Work out the finished part from the listing and answer in its coordinate system (mm). Give positions to 0.01 mm unless a question says otherwise; leave off trailing zeros. Write each loop counter-clockwise with the first axis right and the second up, starting at its lowest first coordinate (ties: lowest second). Pieces come first, ordered by that corner, then holes.
1) Find section D-D (z = 51.5). Determine the outline of the cut face in (x, y).
2) Given pin 1 Ø6.5 at (y, z) = (20, 62.5) entering from +X; pin 2 Ø5 at (x, z) = (-11, 45.5) entering from -Y; pin 3 Ø6 at (y, z) = (25.5, 18.5) entering from +X, each flat-ended and moving along its own axis, determine where each tip first touches the part or whether it passes through.
3) Determine the mould class of faces 1 (the face through (0, 0, 70)), 2 (the face through (-0.195, 31.487, 35.49)), 3 (the face through (-13.366, -0.49, 3.581)) for opening direction X: pulls with the +X half, pulls with the -X half, needs draft (parallel to the pull), parting line crosses it, or undercut.
4) Find section C-C (x = 6). Determine the outline of the cut face in (y, z).
5) Find section A-A (z = 66). Determine the outline of the cut face in (x, y), plus the area to 3 significant figures.
6) Find section B-B (y = -30). Determine the outline of the cut face in (x, z).
7) Straight lines are drawn through the part: probe 1 along Y at (x, z) = (-20, 53); probe 2 along Y at (x, z) = (-12, 62.5); probe 3 along Y at (x, z) = (0.5, 43.5). For each, find the intervals that lie inside material, in ascending order.
```python
from build123d import *

# Parameters (mm, degrees)
F0_R          = 35
F1_DEPTH      = 70
F3_DEPTH      = 35.001
F3_DEPTH_BACK = 35.001
F4_R          = 2.5
F5_DEPTH      = 35.001
F5_DEPTH_BACK = 35.001
F8_R          = 0.5
F9_DEPTH      = 20
F10_R         = 1.5
F11_DEPTH     = 70.0010001


with BuildPart() as f1:
    # F0 (on Top) → F1 (new body)
    with BuildSketch(Plane.XY):
        Circle(F0_R)
    extrude(amount=F1_DEPTH)

    # F2 (on Front) → F3 (cut, two sides)
    with BuildSketch(Plane.XZ) as f3_sk:
        Polygon((-50, 0), (0, 0), (-50, 13.3974596216), align=None)
        Polygon((50, 23.3153829077), (0, 0), (50, 0), align=None)
    extrude(amount=-F3_DEPTH, mode=Mode.SUBTRACT)
    extrude(f3_sk.sketch, amount=F3_DEPTH_BACK, mode=Mode.SUBTRACT)

    # F4 (on Right) → F5 (cut, two sides)
    with BuildSketch(Plane.YZ) as f5_sk:
        with Locations((-20, 62.5)):
            Circle(F4_R)
        with Locations((20, 62.5)):
            Circle(F4_R)
    extrude(amount=-F5_DEPTH, mode=Mode.SUBTRACT)
    extrude(f5_sk.sketch, amount=F5_DEPTH_BACK, mode=Mode.SUBTRACT)

    # F6 (on Front) → F7 (revolve, cut)
    with BuildSketch(Plane.XZ):
        with BuildLine():
            Line((0, 15), (0, 55))
            ThreePointArc((0, 55), (-20, 35), (0, 15))
        make_face()
    revolve(axis=Axis((0, 0, 35), (0, 0, -1)), mode=Mode.SUBTRACT)

    # F8 (on face) → F9 (cut)
    with BuildSketch(Plane.XY.offset(70)):
        with Locations((-20, 20)):
            Circle(F8_R)
        with Locations((-20, -20)):
            Circle(F8_R)
    extrude(amount=-F9_DEPTH, mode=Mode.SUBTRACT)

    # F10 (on face) → F11 (cut, through all)
    with BuildSketch(Plane.XY.offset(70)):
        with Locations((0, 30)):
            Circle(F10_R)
        with Locations((0, -30)):
            Circle(F10_R)
    extrude(amount=-F11_DEPTH, mode=Mode.SUBTRACT)


solid = f1.part
```
Results:
1. outline: circle Ø70 at (0, 0); hole circle Ø1 at (-20, -20); hole circle Ø1 at (-20, 20); hole circle Ø22.61 at (0, 0); hole circle Ø3 at (0, -30); hole circle Ø3 at (0, 30)
2. pin 1: stops at x = 30.73
2. pin 2: stops at y = -33.95
2. pin 3: stops at x = 26.81
3. face 1: needs draft
3. face 2: undercut
3. face 3: pulls with the -X half
4. outline: (-34.48, 2.8) - (34.48, 2.8) - (34.48, 70) - (-34.48, 70) - close; hole circle Ø5 at (-20, 62.5); hole circle Ø38.16 at (0, 35); hole circle Ø5 at (20, 62.5)
5. outline: circle Ø70 at (0, 0); hole circle Ø1 at (-20, -20); hole circle Ø1 at (-20, 20); hole circle Ø3 at (0, -30); hole circle Ø3 at (0, 30)
5. area: 3,830 mm2
6. outline: (-18.03, 4.83) - (-1.5, 0.4) - (-1.5, 70) - (-18.03, 70) - close; (1.5, 0.7) - (18.03, 8.41) - (18.03, 70) - (1.5, 70) - close
7. probe 1: y = -28.72 to -20.5, -19.5 to 19.5, 20.5 to 28.72
7. probe 2: y = -32.88 to -22.5, -17.5 to 17.5, 22.5 to 32.88
7. probe 3: y = -35 to -31.41, -28.59 to -18.1, 18.1 to 28.59, 31.41 to 35
